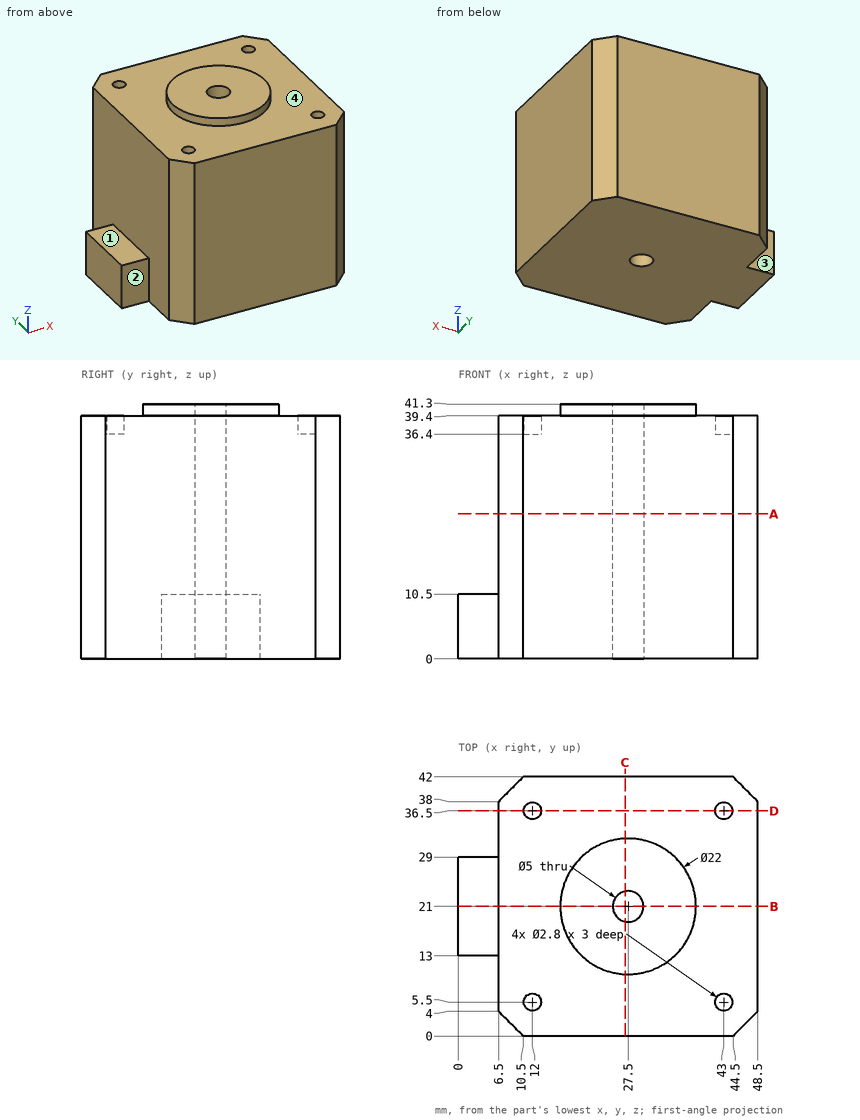
Print and shaded views of the part. All mm, measured from the part's lowest x, y and z. A direction names the side the tool comes from. Give positions to 0.01 mm unless a question says otherwise; leave off trailing zeros. Write each loop counter-clockwise with the first axis right and the second up, starting at its lowest first coordinate (ties: lowest second). Pieces come first, ordered by that corner, then holes. Notation, with made-up numbers: (68.5, 49) -> (114.5, 49) arc R19 ccw to (114.5, 82) -> close; hole circle Ø3 at (56.25, -24.75). An arc over 180 degrees is marked (long way). Write each question's results on one line, items separated by ' | '.
1. Drop flat-ended pins along their axis: P1, Ø7, axis at x = 4.5, z = 5.5, coming from the +Y side; P2, Ø2, axis at x = 3.5, y = 23.5, coming from the +Z side; P3, Ø3, axis at y = 36, z = 34.5, coming from the -X side. Give the stop position or say it passes through.
Geometry check:
P1: y = 39.5 | P2: z = 10.5 | P3: x = 6.5
2. Cut at B-B, the plane y = 21. Write the cut outline in (x, z).
Geometry check:
outline: (0, 0) -> (25, 0) -> (25, 41.3) -> (16.5, 41.3) -> (16.5, 39.4) -> (6.5, 39.4) -> (6.5, 10.5) -> (0, 10.5) -> close; (30, 0) -> (48.5, 0) -> (48.5, 39.4) -> (38.5, 39.4) -> (38.5, 41.3) -> (30, 41.3) -> close
3. Cut at A-A, the plane z = 23.5. Write the cut outline in (x, y), then the cut area to 3 significant figures.
Geometry check:
outline: (6.5, 4) -> (10.5, 0) -> (44.5, 0) -> (48.5, 4) -> (48.5, 38) -> (44.5, 42) -> (10.5, 42) -> (6.5, 38) -> close; hole circle Ø5 at (27.5, 21) | area: 1,710 mm²
4. Cut at C-C, the plane x = 27. Write the cut outline in (y, z), then the cut area to 3 significant figures.
Geometry check:
outline: (0, 0) -> (18.55, 0) -> (18.55, 41.3) -> (10.01, 41.3) -> (10.01, 39.4) -> (0, 39.4) -> close; (23.45, 0) -> (42, 0) -> (42, 39.4) -> (31.99, 39.4) -> (31.99, 41.3) -> (23.45, 41.3) -> close | area: 1,490 mm²
5. Which spindle directions (+Z, -Z, +X, -X, +Y, -Y) get a long thin tool onto all of the face, cutting with end or side? Do the marked faces 1, 2, 3 and 4. Say none if no direction does.
Geometry check:
face 1: +Z, -X, +Y, -Y | face 2: +Z, -Z, -X, -Y | face 3: +Z, -Z, -X, +Y | face 4: +Z
6. Wall check: probe 1 along Y at (x, z) = (12, 37); probe 2 along Z at (x, y) = (40, 3.5); probe 3 along X at (y, z) = (28.5, 37). Give the ranges that are in metal, low to high. Write a range as [from, to].
Geometry check:
probe 1: [0, 4.1], [6.9, 35.1], [37.9, 42] | probe 2: [0, 39.4] | probe 3: [6.5, 48.5]
7. Cut at D-D, the plane y = 36.5. Write the cut outline in (x, z).
Geometry check:
outline: (6.5, 0) -> (48.5, 0) -> (48.5, 39.4) -> (44.4, 39.4) -> (44.4, 36.4) -> (41.6, 36.4) -> (41.6, 39.4) -> (13.4, 39.4) -> (13.4, 36.4) -> (10.6, 36.4) -> (10.6, 39.4) -> (6.5, 39.4) -> close
